Could you check a few things on this model? Use its own coordinates, in mm. A direction names the side the tool comes from. Give positions to 0.01 mm unless a question says otherwise; leave off trailing zeros. Loops run counter-clockwise (first coordinate to the right, second up) from the corner with the lowest first, then second, coordinate; pieces in that order, holes last. Notation, with made-up numbers: M -27,71.5 L 21,71.5 A11 ccw 21,86.5 Z; hole C -35.5,47 d6. An arc over 180 degrees is marked long. Return JSON: item names as keys, results as strings. Group by question number.
1. If we mould it in two halves opening along Y, with no side actions, what happens to faces 4 (the cylindrical face through (-6.247, -0.213, 9.614)), 5 (the flat face through (-1, 11.175, 10)), 6 (the flat face through (-1.3, 5.4, 0))? For each: +Y half, -Y half, draft (parallel to the pull), parting line (faces both ways), or undercut.
2. Please list where these lines run through material, in increasing order: line 1 (Y direction, x = 13, z = 14.5) (3 decimals); line 2 (Z direction, x = -10, y = 8.75); line 3 (X direction, y = 3.5, z = 3.25).
3. If we section it at B-B (y = 7): Write out the boundary of the cut face in (x, z) (3 decimals), plus the area to 3 significant figures.
4. For pin 1 (8 mm diameter, centred on x = -13, y = 5.5, fed in from -Z); pin 2 (3 mm diameter, centred on x = -9.9, z = 10, fed in from -Y); pin 3 (3 mm diameter, centred on x = 9.5, z = 9, fed in from +Y) (3 decimals), each with a flat end and sliding along its axis, tell me the tip position at first contact or that it passes through.
5. If we section it at C-C (y = 0): Write out the boundary of the cut face in (x, z) (3 decimals), plus the area to 3 significant figures.
6. If we section it at D-D (x = 8): Write out the boundary of the cut face in (y, z) (3 decimals).
7. If we section it at A-A (z = 10): State how many separate pieces and enclosed holes the cut face has, plus the area to 3 significant figures.
8. For faces 1 (the flat face through (12, -1.035, 10)), 2 (the cylindrical face through (-14.84, 8.71, 11.55)), 3 (the flat face through (2, 5, 20)), which set-ups out of +Z, -Z, +X, -X, +Y, -Y let a thin tool reach every point of the face, with its end or its side?
```python
from build123d import *

# Parameters (mm, degrees)
F1_DEPTH = 20
F2_R     = 2.675
F3_DEPTH = 20
F2_R_2   = 5.175
F4_DEPTH = 5
F5_SIZE  = 0.5


with BuildPart() as f1:
    # F0 (on Top) → F1 (new body)
    with BuildSketch(Plane.XY):
        with BuildLine():
            Line((14.923915, 11.175), (-17.076085, 11.175))
            Line((-17.076085, 11.175), (-17.076085, -8.825))
            Line((-17.076085, -8.825), (14.923915, -8.825))
            Line((14.923915, -8.825), (14.923915, -1.035))
            Line((14.923915, -1.035), (3.994358, -1.035))
            ThreePointArc((3.994358, -1.035), (-6.251085, 0), (3.994358, 1.035))
            Line((3.994358, 1.035), (14.923915, 1.035))
            Line((14.923915, 1.035), (14.923915, 11.175))
        make_face()
    extrude(amount=F1_DEPTH)

    # F2 (on face) → F3 (cut)
    with BuildSketch(Plane(origin=(0, 11.175, 0), x_dir=(-1, 0, 0), z_dir=(0, 1, 0))):
        with Locations((-7.748915, 10)):
            Circle(F2_R)
        with Locations((9.901085, 10)):
            Circle(F2_R)
    extrude(amount=-F3_DEPTH, mode=Mode.SUBTRACT)

    # F2 (on face) → F4 (cut)
    with BuildSketch(Plane(origin=(0, 11.175, 0), x_dir=(-1, 0, 0), z_dir=(0, 1, 0))):
        with Locations((-7.748915, 10)):
            Circle(F2_R_2)
        with Locations((-7.748915, 10)):
            Circle(F2_R, mode=Mode.SUBTRACT)
        with Locations((9.901085, 10)):
            Circle(F2_R_2)
        with Locations((9.901085, 10)):
            Circle(F2_R, mode=Mode.SUBTRACT)
    extrude(amount=-F4_DEPTH, mode=Mode.SUBTRACT)

    # F5
    f5_edges = [f1.edges().sort_by_distance(p)[0] for p in [
        (14.923915, -1.035, 10),
        (-17.076085, 1.175, 20),
        (-1.076085, 11.175, 20),
        (-17.076085, 11.175, 10),
        (14.923915, 11.175, 10),
        (14.923915, 6.105, 20),
        (14.923915, -4.93, 20),
        (-6.251085, 0, 20),
        (14.923915, 1.035, 10),
        (-1.076085, 11.175, 0),
    ]]
    chamfer(f5_edges, length=F5_SIZE)


solid = f1.part
```
Answer:
{
 "1": {"face 4": "undercut", "face 5": "+Y half", "face 6": "draft"},
 "2": {"line 1": "y = -8.825 to -1.035, 1.035 to 11.175", "line 2": "z = 0 to 4.83, 15.17 to 20", "line 3": "x = -17.08 to -4.89, 2.74 to 14.92"},
 "3": {"outline": "M -17.076,0 L 14.924,0 L 14.924,19.5 L 14.424,20 L -16.576,20 L -17.076,19.5 Z; hole C -9.901,10 d10.35; hole C 7.749,10 d10.35", "area": "471 mm²"},
 "4": {"pin 1": "stops at z = 0", "pin 2": "passes through", "pin 3": "stops at y = 6.175"},
 "5": {"outline": "M -17.076,0 L -6.251,0 L -6.251,19.5 L -6.751,20 L -16.576,20 L -17.076,19.5 Z; hole C -9.901,10 d5.35", "area": "194 mm²"},
 "6": {"outline": "M -8.825,0 L -1.035,0 L -1.035,7.337 L -8.825,7.337 Z; M -8.825,12.663 L -1.035,12.663 L -1.035,20 L -8.825,20 Z; M 1.035,0 L 10.675,0 L 11.175,0.5 L 11.175,4.831 L 6.175,4.831 L 6.175,7.337 L 1.035,7.337 Z; M 1.035,12.663 L 6.175,12.663 L 6.175,15.169 L 11.175,15.169 L 11.175,19.5 L 10.675,20 L 1.035,20 Z"},
 "7": {"separate pieces": "4", "enclosed holes": "0", "area": "280 mm²"},
 "8": {"face 1": "+Z, -Z, +X", "face 2": "+Y", "face 3": "+Z, +X, -X, +Y, -Y"}
}
